Check sheet for the drawn part. Datum: minimum x, y, z corner. Units: mm. A direction names the side the tool comes from. Give positions to 0.01 mm unless a question says otherwise; leave off trailing zeros. Write each loop counter-clockwise with the first axis right and the second up, starting at its lowest first coordinate (ties: lowest second). Pieces come first, ordered by that corner, then holes. Notation, with made-up numbers: (-33.5, -13) - (-27.5, -13) arc R11 ccw to (-27.5, 4) - close; hole circle Ø8 at (34, -7.5). An arc over 180 degrees is marked (long way). Answer as a JSON object with one key per item and string values. Group by question number.
Item 1: Sectioned sample at B-B, the plane x = 15.75. Record the boundary of the cut face in (y, z), and give its area (3 significant figures).
Item 2: Sectioned sample at A-A, the plane y = 2.75. Record the boundary of the cut face in (x, z), and give its area (3 significant figures).
Item 3: Sectioned sample at C-C, the plane z = 6. Record the boundary of the cut face in (x, y).
Item 4: Tool access check on the marked faces 1 and 2. Record the directions out of +Z, -Z, +X, -X, +Y, -Y that give a thin tool (end or side, any length) a straight path to the whole face; none if there is none.
Item 5: Sectioned sample at D-D, the plane x = 7. Record the boundary of the cut face in (y, z), and give its area (3 significant figures).
Item 6: Go/stop test with flat-tipped pins: pin 1 (1.8 mm diameter, centred on y = 12.75, z = 26, fed in from -X); pin 2 (6 mm diameter, centred on y = 8, z = 13.5, fed in from -X). Record where each tip stops, or that it passes through.
Item 7: Scan lines: line 1 along Z through (x, y) = (15.4, 12.75); line 2 along Z through (x, y) = (7.5, 20.8); line 3 along X through (y, z) = (17.5, 20.75). Record each from-to range of solid material in increasing order. Write a range as [from, to].
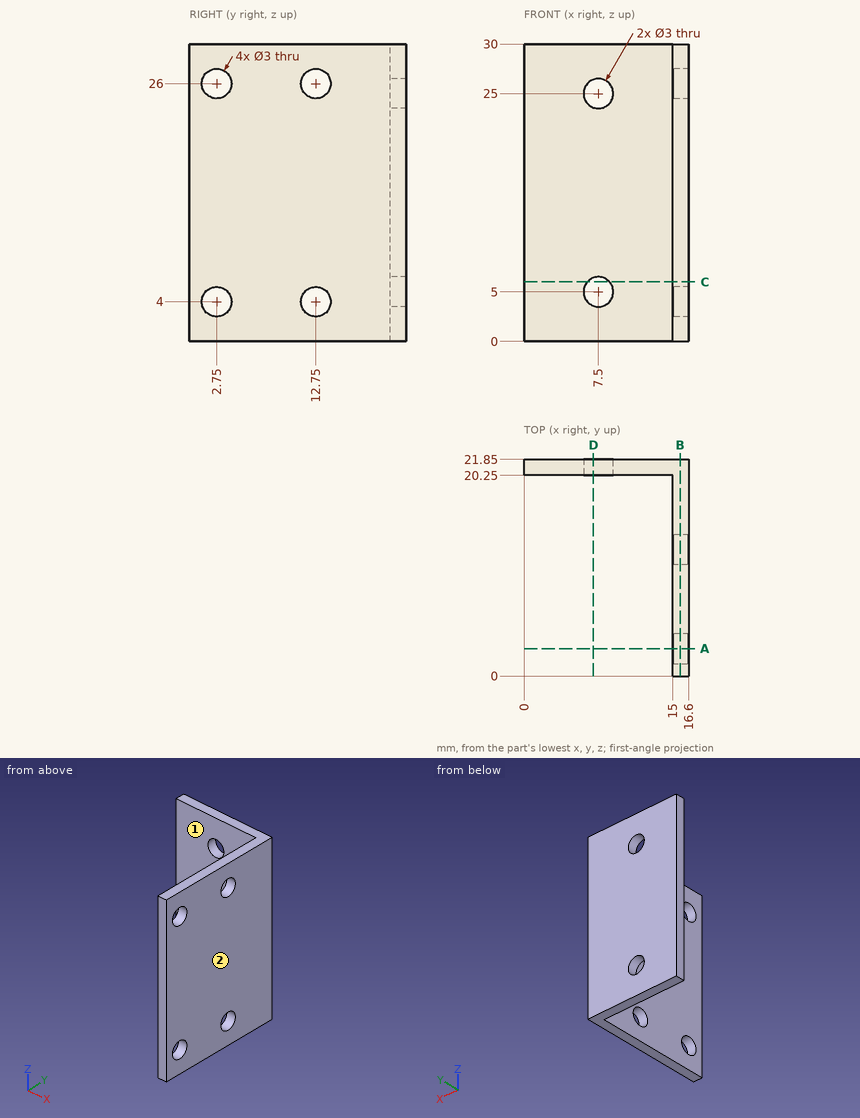
Geometry check:
{
 "1": {"outline": "(0, 0) - (21.85, 0) - (21.85, 30) - (0, 30) - close; hole circle Ø3 at (2.75, 4); hole circle Ø3 at (2.75, 26); hole circle Ø3 at (12.75, 4); hole circle Ø3 at (12.75, 26)", "area": "627 mm^2"},
 "2": {"outline": "(15, 0) - (16.6, 0) - (16.6, 2.5) - (15, 2.5) - close; (15, 5.5) - (16.6, 5.5) - (16.6, 24.5) - (15, 24.5) - close; (15, 27.5) - (16.6, 27.5) - (16.6, 30) - (15, 30) - close", "area": "38.4 mm^2"},
 "3": {"outline": "(0, 20.25) - (6.38, 20.25) - (6.38, 21.85) - (0, 21.85) - close; (8.62, 20.25) - (15, 20.25) - (15, 0) - (16.6, 0) - (16.6, 21.85) - (8.62, 21.85) - close"},
 "4": {"face 1": "+Z, -Z, -X, -Y", "face 2": "+Z, -Z, +X, +Y, -Y"},
 "5": {"outline": "(20.25, 0) - (21.85, 0) - (21.85, 3.59) - (20.25, 3.59) - close; (20.25, 6.41) - (21.85, 6.41) - (21.85, 23.59) - (20.25, 23.59) - close; (20.25, 26.41) - (21.85, 26.41) - (21.85, 30) - (20.25, 30) - close", "area": "38.9 mm^2"},
 "6": {"pin 1": "through", "pin 2": "x = 15"},
 "7": {"line 1": "[0, 2.5], [5.5, 24.5], [27.5, 30]", "line 2": "[0, 3.5], [6.5, 23.5], [26.5, 30]", "line 3": "[15, 16.6]"}
}
